CAD build for the part. Positions are in the model's coordinates, mm. Coordinates: 2 decimals unless noted, no trailing zeros. Order: outer loops, then holes, each group sorted by start corner. A loop starts at its lowest first (then second) coordinate and runs counter-clockwise, first axis right, second up. Notation, with made-up numbers: M 65,47 L 76,47 A15 cw 76,55 Z; hole C 2.5,64.5 d7. An arc over 180 degrees is marked long. One line per item, written item: value.
from build123d import *

# Parameters (mm, degrees)
SKETCH1_W           = 100
SKETCH1_H           = 130
SKETCH1_R           = 2.5
BOSS_EXTRUDE1_DEPTH = 6
FILLET1_R           = 3
SCALE1_SCALE        = 7.5


with BuildPart() as part:
    # Sketch1 → Boss-Extrude1 (new body)
    with BuildSketch(Plane(origin=(0, 0, 0), x_dir=(1, 0, 0), z_dir=(0, 1, 0))):
        with Locations((40, 55)):
            Rectangle(SKETCH1_W, SKETCH1_H)
        Circle(SKETCH1_R, mode=Mode.SUBTRACT)
        with Locations((80, 0)):
            Circle(SKETCH1_R, mode=Mode.SUBTRACT)
        with Locations((0, 80)):
            Circle(SKETCH1_R, mode=Mode.SUBTRACT)
        with Locations((80, 80)):
            Circle(SKETCH1_R, mode=Mode.SUBTRACT)
        with Locations((22, 22)):
            Circle(SKETCH1_R, mode=Mode.SUBTRACT)
        with Locations((58, 22)):
            Circle(SKETCH1_R, mode=Mode.SUBTRACT)
        with Locations((22, 54)):
            Circle(SKETCH1_R, mode=Mode.SUBTRACT)
        with Locations((58, 54)):
            Circle(SKETCH1_R, mode=Mode.SUBTRACT)
    extrude(amount=BOSS_EXTRUDE1_DEPTH)

    # Fillet1
    fillet1_edges = [part.edges().sort_by_distance(p)[0] for p in [
        (90, 3, 10),
        (-10, 3, 10),
    ]]
    fillet(fillet1_edges, radius=FILLET1_R)


with BuildPart() as part_1:
    # Scale1: scaled about (40, 3, -55.215106893)
    add(part.part.scale(SCALE1_SCALE).moved(Location((-260, -19.5, 358.898194805))))


solid = part_1.part
Q1. Mould opens along X. For faces 1 (the face through (415, 3, -58)), 2 (the face through (-264.065, 2.685, 377.202)), 3 (the face through (35, -19.5, -60)) say: released by +X, released by -X, zero draft, split by the parting line, or undercut.
Recorded:
face 1: released by +X
face 2: undercut
face 3: zero draft
Q2. Slice it at A-A (x = -95). List the corners of the cut face in (y, z).
Recorded:
outline: M -19.5,-541.1 L 25.5,-541.1 L 25.5,-64.85 L -19.5,-64.85 Z; M -19.5,-27.35 L 25.5,-27.35 L 25.5,175.15 L -19.5,175.15 Z; M -19.5,212.65 L 25.5,212.65 L 25.5,433.9 L -19.5,433.9 Z
Q3. Drill centre lines: line 1 along Z through (x, y) = (175, -3); line 2 along Z through (x, y) = (340, 1); line 3 along X through (y, z) = (-9, -253). Where is each one in solid material? Low to high.
Recorded:
line 1: z = -541.1 to -64.85, -27.35 to 175.15, 212.65 to 433.9
line 2: z = -541.1 to -259.85, -222.35 to 340.15, 377.65 to 433.9
line 3: x = -335 to -274.49, -245.51 to 325.51, 354.49 to 415
